Autodesk Inventor part; units mm, degrees
ref_plane "YZ Plane" through (0, 0, 0) normal (1, 0, 0) x (0, 1, 0)
ref_plane "XZ Plane" through (0, 0, 0) normal (0, 1, 0) x (-1, 0, 0)
ref_plane "XY Plane" through (0, 0, 0) normal (0, 0, 1) x (1, 0, 0)
sketch "Sketch1" plane through (0, 0, 0) normal (0, 0, 1) x (1, 0, 0)
  line L0 (20, 0) -> (20, 15)
  line L1 (20, 15) -> (0, 15)
  line L2 (0, 15) -> (0, 0)
  circle A0 centre (10, 0) radius 10
  circle A1 centre (10, 0) radius 2
  line L3 (0, 0) -> (8, 0)
  line L4 (12, 0) -> (20, 0)
  dimension "d3" = 20
  dimension "d4" = 15
  dimension "d5" = 4
extrude "Extrusion1" add sketch "Sketch1" along normal blind 3 contours A0 L2 L1 L0 | L4 A1 L3 A0 | A0 L3 A1 L4
sketch "Sketch3" plane through (0, 0, 3) normal (0, 0, 1) x (1, 0, 0)
  circle A0 centre (10, 0) radius 2
  circle A1 centre (10, 0) radius 6
  line L0 (0, 15) -> (0, 0)
  arc A2 (0, 0) -> (20, 0) centre (10, 0) ccw
  line L1 (0, 15) -> (20, 15)
  line L2 (20, 15) -> (20, 0)
  line L3 (0, 0) -> (0, 15)
  dimension "d8" = 12
extrude "Extrusion2" add sketch "Sketch3" along normal blind 8 contours L1 L2 A2 L0
sketch "Sketch4" plane through (0, 0, 11) normal (0, 0, 1) x (1, 0, 0)
  line L0 (0, 15) -> (20, 15)
  line L1 (20, 15) -> (20, 10)
  line L2 (20, 10) -> (0, 10)
  line L3 (0, 10) -> (0, 15)
  line L4 (20, 15) -> (0, 15)
  point P0 (0, 0)
  dimension "d11" = 20
  dimension "d12" = 5
extrude "Extrusion3" add sketch "Sketch4" along normal blind 4
sketch "Sketch5" plane through (0, 10, 11) normal (0, -1, 0) x (1, 0, 0)
  circle A0 centre (5, 1.6) radius 1.6
  circle A1 centre (15, 1.6) radius 1.6
  line L0 (0, 0) -> (0, 4)
  line L1 (20, 0) -> (20, 4)
  line L2 (0, 4) -> (20, 4)
  line L3 (20, 0) -> (0, 0)
  line L4 (3.4, 1.6) -> (3.4, 4)
  line L5 (13.4, 1.6) -> (13.4, 4)
  line L6 (16.6, 1.6) -> (16.6, 4)
  line L7 (6.6, 1.6) -> (6.6, 4)
  point P0 (0, -11)
  dimension "d15" = 3.2
  dimension "d16" = 3.2
  dimension "d21" = 5
  dimension "d23" = 5
extrude "Extrusion4" cut sketch "Sketch5" against normal through all contours A0 | A0 L4 L2 L7 | A1 | L2 L6 A1 L5
fillet "Fillet2" radius 2 5 edges at (0, 10, 13) (10, -10, 11) (20, 5, 11) (0, 5, 11) (20, 10, 13)
properties part number "clip"
Can you work these out from the model? Positions are in its coordinate system, mm. A direction names the side the tool comes from. Round coordinates to 2 decimals unless told otherwise and drop trailing zeros. Loops run counter-clockwise (first coordinate to the right, second up) from the corner with the lowest first, then second, coordinate; pieces in that order, holes last. Notation, with made-up numbers: M 7,15.5 L 44,15.5 A18 cw 44,48.5 Z; hole C 34,-15.75 d8. An arc over 180 degrees is marked long. Answer as a JSON object with one key per item and string values. Group by question number.
Q1. On a 3-axis mill with a long thin cutter (end or side, diameter ignored), from which of +Z, -Z, +X, -X, +Y, -Y can I reach the whole of each face in a straight line? I mean faces 1 (the cylindrical face through (0.57, 10.6, 12.71)), 2 (the flat face through (13.4, 12, 14)), 3 (the flat face through (6, 5, 11)). Say none if no direction works.
Q2. Please list where these lines run through material, in increasing order: L1, parallel to X at y = 0, z = 0.8; L2, parallel to Y at x = 10, z = 1.15; L3, parallel to Y at x = 10, z = 5.5.
Q3. Will these pins go through, and if not, where does the flat tip stop? pin 1 (0.9 mm diameter, centred on x = 16, z = 14, fed in from -Y); pin 2 (2.5 mm diameter, centred on y = 13.5, z = 14, fed in from -X); pin 3 (5 mm diameter, centred on x = 10, y = 0, fed in from +Z); pin 4 (1.5 mm diameter, centred on x = 3, z = 12, fed in from -Y).
Q4. Imagine slicing it at D-D, the plane y = 5.25. Please give me the cut outline in (x, z).
Q5. Imagine slicing it at B-B, the plane z = 13.25. Please give me the cut outline in (x, y), then the cut area to 3 significant figures.
Q6. Imagine slicing it at C-C, the plane z = 8.25. Please give me the cut outline in (x, y), then the cut area to 3 significant figures.
Q7. Imagine slicing it at A-A, the plane x = 10. Please give me the cut outline in (y, z), then the cut area to 3 significant figures.
Q8. We'd pull the mould along X, two halves only. Please class faces 4 (the flat face through (10, 10, 13)), 5 (the cylindrical face through (19.4, 6.08, 10.43)), 6 (the flat face through (3.4, 12, 14)): +X half, -X half, draft (parallel to the pull), parting line (faces both ways), or undercut.
Findings:
{
 "1": {"face 1": "+Z, -X, -Y", "face 2": "+Z, +Y, -Y", "face 3": "+Z, +X, -X, -Y"},
 "2": {"L1": "x = 0 to 8, 12 to 20", "L2": "y = -10 to -2, 2 to 15", "L3": "y = -10 to -6, 6 to 15"},
 "3": {"pin 1": "passes through", "pin 2": "stops at x = 0", "pin 3": "stops at z = 3", "pin 4": "stops at y = 10"},
 "4": {"outline": "M 0,0 L 20,0 L 20,9 A2 ccw 18,11 L 12.9,11 L 12.9,3 L 7.1,3 L 7.1,11 L 2,11 A2 ccw 0,9 Z"},
 "5": {"outline": "M 0,12 A2 ccw 2,10 L 3.4,10 L 3.4,15 L 0,15 Z; M 6.6,10 L 13.4,10 L 13.4,15 L 6.6,15 Z; M 16.6,10 L 18,10 A2 ccw 20,12 L 20,15 L 16.6,15 Z", "area": "66.3 mm2"},
 "6": {"outline": "M 0,0 A10 ccw 20,0 L 20,15 L 0,15 Z; hole C 10,0 d12", "area": "344 mm2"},
 "7": {"outline": "M -10,0 L -2,0 L -2,3 L -6,3 L -6,11 L -8,11 A2 ccw -10,9 Z; M 2,0 L 15,0 L 15,15 L 10,15 L 10,11 L 6,11 L 6,3 L 2,3 Z", "area": "186 mm2"},
 "8": {"face 4": "draft", "face 5": "+X half", "face 6": "undercut"}
}
